```python
from build123d import *

# Parameters (mm, degrees)
ESBO_O1_R                = 5
RESSALTO_EXTRUS_O1_DEPTH = 1250
ESBO_O4_W                = 0.75
ESBO_O4_H                = 0.5
ESBO_O4_W_2              = 0.5
ESBO_O4_H_2              = 0.75
CORTE_EXTRUS_O1_DEPTH    = 1250


with BuildPart() as part:
    # Esboço1 → Ressalto-extrusão1 (new body)
    with BuildSketch(Plane(origin=(0, 0, 0), x_dir=(1, 0, 0), z_dir=(0, 1, 0))):
        with BuildLine():
            Line((-18, -20), (-5, -20))
            Line((-5, -20), (-5, -18))
            Line((-5, -18), (-10.5, -18))
            Line((-10.5, -18), (-10.5, -11.206655676))
            Line((-10.5, -11.206655676), (-4.583792723, -5.2904484))
            ThreePointArc((-4.583792723, -5.2904484), (0, -7), (4.583792723, -5.2904484))
            Line((4.583792723, -5.2904484), (10.5, -11.206655676))
            Line((10.5, -11.206655676), (10.5, -18))
            Line((10.5, -18), (5, -18))
            Line((5, -18), (5, -20))
            Line((5, -20), (18, -20))
            ThreePointArc((18, -20), (19.414213562, -19.414213562), (20, -18))
            Line((20, -18), (20, -5))
            Line((20, -5), (18, -5))
            Line((18, -5), (18, -10.5))
            Line((18, -10.5), (11.206655676, -10.5))
            Line((11.206655676, -10.5), (5.2904484, -4.583792723))
            ThreePointArc((5.2904484, -4.583792723), (7, 0), (5.2904484, 4.583792723))
            Line((5.2904484, 4.583792723), (11.206655676, 10.5))
            Line((11.206655676, 10.5), (18, 10.5))
            Line((18, 10.5), (18, 5))
            Line((18, 5), (20, 5))
            Line((20, 5), (20, 18))
            ThreePointArc((20, 18), (19.414213562, 19.414213562), (18, 20))
            Line((18, 20), (5, 20))
            Line((5, 20), (5, 18))
            Line((5, 18), (10.5, 18))
            Line((10.5, 18), (10.5, 11.206655676))
            Line((10.5, 11.206655676), (4.583792723, 5.2904484))
            ThreePointArc((4.583792723, 5.2904484), (0, 7), (-4.583792723, 5.2904484))
            Line((-4.583792723, 5.2904484), (-10.5, 11.206655676))
            Line((-10.5, 11.206655676), (-10.5, 18))
            Line((-10.5, 18), (-5, 18))
            Line((-5, 18), (-5, 20))
            Line((-5, 20), (-18, 20))
            ThreePointArc((-18, 20), (-19.414213562, 19.414213562), (-20, 18))
            Line((-20, 18), (-20, 5))
            Line((-20, 5), (-18, 5))
            Line((-18, 5), (-18, 10.5))
            Line((-18, 10.5), (-11.206655676, 10.5))
            Line((-11.206655676, 10.5), (-5.2904484, 4.583792723))
            ThreePointArc((-5.2904484, 4.583792723), (-7, 0), (-5.2904484, -4.583792723))
            Line((-5.2904484, -4.583792723), (-11.206655676, -10.5))
            Line((-11.206655676, -10.5), (-18, -10.5))
            Line((-18, -10.5), (-18, -5))
            Line((-18, -5), (-20, -5))
            Line((-20, -5), (-20, -18))
            ThreePointArc((-20, -18), (-19.414213562, -19.414213562), (-18, -20))
        make_face()
        with Locations(Location((0, 0, 0), (0, 0, 270))):
            Circle(ESBO_O1_R, mode=Mode.SUBTRACT)
        with BuildLine():
            Line((-19.25, 5.75), (-18.75, 5.75))
            Line((-18.75, 5.75), (-18.75, 11.25))
            Line((-18.75, 11.25), (-11.25, 11.25))
            Line((-11.25, 11.25), (-11.25, 18.75))
            Line((-11.25, 18.75), (-5.75, 18.75))
            Line((-5.75, 18.75), (-5.75, 19.25))
            Line((-5.75, 19.25), (-17.469669914, 19.25))
            ThreePointArc((-17.469669914, 19.25), (-18.728553391, 18.728553391), (-19.25, 17.469669914))
            Line((-19.25, 17.469669914), (-19.25, 5.75))
        make_face(mode=Mode.SUBTRACT)
        with BuildLine():
            Line((19.25, 5.75), (19.25, 17.469669914))
            ThreePointArc((19.25, 17.469669914), (18.728553391, 18.728553391), (17.469669914, 19.25))
            Line((17.469669914, 19.25), (5.75, 19.25))
            Line((5.75, 19.25), (5.75, 18.75))
            Line((5.75, 18.75), (11.25, 18.75))
            Line((11.25, 18.75), (11.25, 11.25))
            Line((11.25, 11.25), (18.75, 11.25))
            Line((18.75, 11.25), (18.75, 5.75))
            Line((18.75, 5.75), (19.25, 5.75))
        make_face(mode=Mode.SUBTRACT)
        with BuildLine():
            Line((19.25, -5.75), (18.75, -5.75))
            Line((18.75, -5.75), (18.75, -11.25))
            Line((18.75, -11.25), (11.25, -11.25))
            Line((11.25, -11.25), (11.25, -18.75))
            Line((11.25, -18.75), (5.75, -18.75))
            Line((5.75, -18.75), (5.75, -19.25))
            Line((5.75, -19.25), (17.469669914, -19.25))
            ThreePointArc((17.469669914, -19.25), (18.728553391, -18.728553391), (19.25, -17.469669914))
            Line((19.25, -17.469669914), (19.25, -5.75))
        make_face(mode=Mode.SUBTRACT)
        with BuildLine():
            Line((-19.25, -5.75), (-19.25, -17.469669914))
            ThreePointArc((-19.25, -17.469669914), (-18.728553391, -18.728553391), (-17.469669914, -19.25))
            Line((-17.469669914, -19.25), (-5.75, -19.25))
            Line((-5.75, -19.25), (-5.75, -18.75))
            Line((-5.75, -18.75), (-11.25, -18.75))
            Line((-11.25, -18.75), (-11.25, -11.25))
            Line((-11.25, -11.25), (-18.75, -11.25))
            Line((-18.75, -11.25), (-18.75, -5.75))
            Line((-18.75, -5.75), (-19.25, -5.75))
        make_face(mode=Mode.SUBTRACT)
    extrude(amount=RESSALTO_EXTRUS_O1_DEPTH)

    # Esboço4 → Corte-extrusão1 (cut)
    with BuildSketch(Plane(origin=(0, 1250, 0), x_dir=(1, 0, 0), z_dir=(0, 1, 0))):
        with Locations((-5.375, 19.75)):
            Rectangle(ESBO_O4_W, ESBO_O4_H)
        with Locations((19.75, 5.375)):
            Rectangle(ESBO_O4_W_2, ESBO_O4_H_2)
        with Locations((-19.75, 5.375)):
            Rectangle(ESBO_O4_W_2, ESBO_O4_H_2)
        with Locations((5.375, 19.75)):
            Rectangle(ESBO_O4_W, ESBO_O4_H)
        with Locations((5.375, -19.75)):
            Rectangle(ESBO_O4_W, ESBO_O4_H)
        with Locations((19.75, -5.375)):
            Rectangle(ESBO_O4_W_2, ESBO_O4_H_2)
        with Locations((-19.75, -5.375)):
            Rectangle(ESBO_O4_W_2, ESBO_O4_H_2)
        with Locations((-5.375, -19.75)):
            Rectangle(ESBO_O4_W, ESBO_O4_H)
    extrude(amount=-CORTE_EXTRUS_O1_DEPTH, mode=Mode.SUBTRACT)


solid = part.part
```
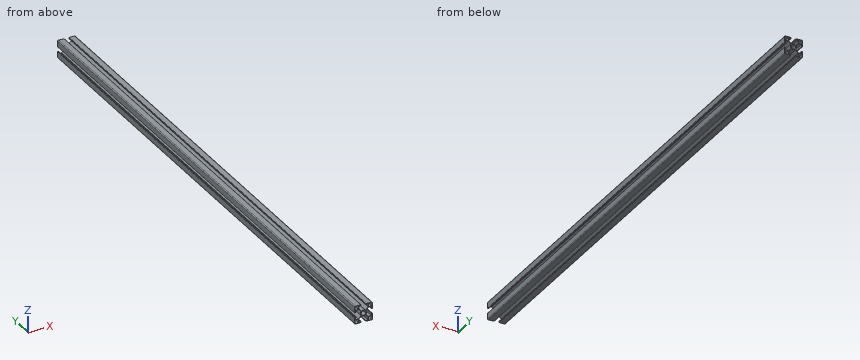
Verification items for the finished model (mm, model axes). Coordinates: 2 decimals unless noted, no trailing zeros. Return JSON: item names as keys, results as strings.
1. Thickness scan on L1, parallel to Z at x = 13, y = 703; L2, parallel to Z at x = 18.5, y = 1075. Record the ranges inside material, lowest first.
Established:
{"L1": "z = -20 to -19.25, -11.25 to -10.5, 10.5 to 11.25, 19.25 to 20", "L2": "z = -19.94 to -18.92, -11.25 to -5, 5 to 11.25, 18.92 to 19.94"}
2. Go/stop test with flat-tipped pins: pin 1 (1.5 mm diameter, centred on x = -2.5, z = -1.5, fed in from -Y); pin 2 (1.5 mm diameter, centred on y = 937, z = -2.5, fed in from -X). Record where each tip stops, or that it passes through.
Established:
{"pin 1": "passes through", "pin 2": "stops at x = -6.78"}
3. Section check A-A, the plane y = 916. Count the separate pieces of the cut face and the enclosed holes in it, then the cut area to 3 significant figures.
Established:
{"separate pieces": "1", "enclosed holes": "5", "area": "275 mm2"}
